```python
from build123d import *

# Parameters (mm, degrees)
F0_R     = 1.5
F1_DEPTH = 5
F2_W     = 39.6
F2_H     = 20
F3_DEPTH = 5
F2_W_2   = 5
F4_DEPTH = 6
F5_ANGLE = 90


with BuildPart() as f1:
    # F0 (on Top) → F1 (new body)
    with BuildSketch(Plane.XY):
        Circle(F0_R)
    extrude(amount=-F1_DEPTH)

    # F2 (on Top) → F3 (join)
    with BuildSketch(Plane.XY):
        Rectangle(F2_W, F2_H)
    extrude(amount=F3_DEPTH)

    # F2 (on Top) → F4 (join)
    with BuildSketch(Plane.XY):
        with Locations((-22.3, 0)):
            Rectangle(F2_W_2, F2_H)
        with Locations((22.3, 0)):
            Rectangle(F2_W_2, F2_H)
    extrude(amount=F4_DEPTH)


with BuildPart() as f1_1:
    # F5: moved
    add(f1.part.rotate(Axis((0, 0, -5), (0, 0, 1)), F5_ANGLE))


solid = f1_1.part
```
Check sheet for the modelled part. Datum: model origin and axes. Units: mm. A direction names the side the tool comes from. Give positions to 0.01 mm unless a question says otherwise; leave off trailing zeros. Loops run counter-clockwise (first coordinate to the right, second up) from the corner with the lowest first, then second, coordinate; pieces in that order, holes last. Notation, with made-up numbers: M 49,58.5 L 76,58.5 A23 ccw 76,92.5 Z; hole C 76.5,-39.75 d7. An arc over 180 degrees is marked long. Answer in a Markdown table with one row per item.
1) Cross-section at B-B (x = 0). Enter the section's corners in (y, z), plus the area to 3 significant figures.
Solutions:
| item | result |
|---|---|
| outline | M -24.8,0 L -1.5,0 L -1.5,-5 L 1.5,-5 L 1.5,0 L 24.8,0 L 24.8,6 L 19.8,6 L 19.8,5 L -19.8,5 L -19.8,6 L -24.8,6 Z |
| area | 273 mm^2 |
2) Thickness scan on line 1 (Y direction, x = 0.5, z = 5.25); line 2 (Z direction, x = 4, y = 10.5); line 3 (Y direction, x = 1.25, z = -0.25). Record the ranges inside material, lowest first.
Solutions:
| item | result |
|---|---|
| line 1 | y = -24.8 to -19.8, 19.8 to 24.8 |
| line 2 | z = 0 to 5 |
| line 3 | y = -0.83 to 0.83 |
3) Depth check by flat-ended pin: pin 1 (10 mm diameter, centred on x = 6, y = 3, fed in from -Z). Enter the tip coordinate at first touch or a pass-through.
Solutions:
| item | result |
|---|---|
| pin 1 | stops at z = 0 |
4) Cross-section at A-A (y = 0). Enter the section's corners in (x, z), plus the area to 3 significant figures.
Solutions:
| item | result |
|---|---|
| outline | M -10,0 L -1.5,0 L -1.5,-5 L 1.5,-5 L 1.5,0 L 10,0 L 10,5 L -10,5 Z |
| area | 115 mm^2 |
5) Cross-section at C-C (z = -1.5). Enter the section's corners in (x, y), plus the area to 3 significant figures.
Solutions:
| item | result |
|---|---|
| outline | C 0,0 d3 |
| area | 7.07 mm^2 |
6) Mould release check, pull along Y, two halves, no side actions. Record for faces 1 (the face through (0, 0, 5)), 2 (the face through (0, -22, 6)), 3 (the face through (0, -24.8, 3)): released by +Y, released by -Y, zero draft, split by the parting line, or undercut.
Solutions:
| item | result |
|---|---|
| face 1 | undercut |
| face 2 | zero draft |
| face 3 | released by -Y |
7) Cross-section at D-D (x = -7). Enter the section's corners in (y, z), plus the area to 3 significant figures.
Solutions:
| item | result |
|---|---|
| outline | M -24.8,0 L 24.8,0 L 24.8,6 L 19.8,6 L 19.8,5 L -19.8,5 L -19.8,6 L -24.8,6 Z |
| area | 258 mm^2 |
8) Tool access check on faces 4 (the face through (0.1, 19.8, 5.5)), 5 (the face through (-0.45, 1.43, -2.46)), 6 (the face through (0, 24.8, 3)). Record the directions out of +Z, -Z, +X, -X, +Y, -Y that give a thin tool (end or side, any length) a straight path to the whole face; none if there is none.
Solutions:
| item | result |
|---|---|
| face 4 | +Z, +X, -X |
| face 5 | -Z |
| face 6 | +Z, -Z, +X, -X, +Y |
